Autodesk Fusion 360 part; units mm, degrees
sketch "Sketch1" plane through (0, 0, 0) normal (0, 0, 1) x (1, 0, 0)
  circle A0 centre (0, 0) radius 3.6
  dimension "d1" = 7.2
extrude "Extrude1" add sketch "Sketch1" along normal blind 50
sketch "Sketch2" plane through (0, 0, 50) normal (0, 0, 1) x (-1, 0, 0)
  circle A0 centre (0, 0) radius 3.6
  circle A1 centre (0, 0) radius 2
  dimension "d4" = 4
extrude "Extrude2" cut sketch "Sketch2" against normal blind 6.7 contours A1
sketch "Sketch3" plane through (0, 0, 0) normal (0, 0, -1) x (1, 0, 0)
  circle A0 centre (0, 0) radius 3.6
  circle A1 centre (0, 0) radius 2
  dimension "d7" = 4
extrude "Extrude3" cut sketch "Sketch3" against normal blind 6.7 contours A1
Could you check a few things on this model? Use its own coordinates, in mm. A direction names the side the tool comes from. Give positions to 0.01 mm unless a question says otherwise; leave off trailing zeros. Loops run counter-clockwise (first coordinate to the right, second up) from the corner with the lowest first, then second, coordinate; pieces in that order, holes last. Notation, with made-up numbers: (70.5, 60.25) -> (88.5, 60.25) arc R22 cw to (88.5, 87.25) -> close; hole circle Ø11 at (-15.75, 85.25). An arc over 180 degrees is marked (long way). Answer as CSV lines item,"result". Start each with the question number.
(1) I'm going to push flat-ended pins straight in: pin 1 Ø3 at (x, z) = (-2, 18.5) entering from +Y; pin 2 Ø1.5 at (y, z) = (-2.5, 14.5) entering from -X; pin 3 Ø4 at (x, y) = (-2.5, -0.5) entering from -Z; pin 4 Ø2.5 at (x, y) = (0, 0) entering from +Z. Where does each tip first touch, or does it pass through?
(2) If we section it at C-C on z = 24.5: Write out the boundary of the cut face in (x, y), then the cut area to 3 significant figures.
(3) We'd pull the mould along X, two halves only. Please class faces 1 (the cylindrical face through (3.434, -1.081, 24.65)), 2 (the flat face through (0, 0, 43.3)), 3 (the flat face through (2, -2, 50)): released by +X, released by -X, zero draft, split by the parting line, or undercut.
(4) If we section it at D-D on x = -2.5: Write out the boundary of the cut face in (y, z), then the cut area to 3 significant figures.
(5) If we section it at A-A on y = 0: Write out the boundary of the cut face in (x, z).
(6) I need wall thicknesses on probe 1 along Y at (x, z) = (0, 4.5); probe 2 along X at (y, z) = (0.25, 12); probe 3 along Z at (x, y) = (-1.25, -1.25). Which ranges of each line are inside material? Lowest first, please.
(7) Which directions (+Z, -Z, +X, -X, +Y, -Y) give clear straight access to the entire face, cutting with the end or side of a thin tool? Please do faces 4 (the flat face through (0, 0, 6.7)), 5 (the flat face through (2, -2, 0)), 6 (the cylindrical face through (0, 2, 47)).
Computed:
1,pin 1,"stops at y = 3.57"
1,pin 2,"stops at x = -3.15"
1,pin 3,"stops at z = 0"
1,pin 4,"stops at z = 43.3"
2,outline,"circle Ø7.2 at (0, 0)"
2,area,"40.7 mm2"
3,face 1,"split by the parting line"
3,face 2,"undercut"
3,face 3,"zero draft"
4,outline,"(-2.59, 0) -> (2.59, 0) -> (2.59, 50) -> (-2.59, 50) -> close"
4,area,"259 mm2"
5,outline,"(-3.6, 0) -> (-2, 0) -> (-2, 6.7) -> (2, 6.7) -> (2, 0) -> (3.6, 0) -> (3.6, 50) -> (2, 50) -> (2, 43.3) -> (-2, 43.3) -> (-2, 50) -> (-3.6, 50) -> close"
6,probe 1,"y = -3.6 to -2, 2 to 3.6"
6,probe 2,"x = -3.59 to 3.59"
6,probe 3,"z = 6.7 to 43.3"
7,face 4,"-Z"
7,face 5,"-Z, +X, -X, +Y, -Y"
7,face 6,"+Z"
